```python
from build123d import *

# Parameters (mm, degrees)
F1_DEPTH = 20
F3_DEPTH = 0.2
F5_DEPTH = 20.001


with BuildPart() as f1:
    # F0 (on Top) → F1 (new body)
    with BuildSketch(Plane.XY):
        with BuildLine():
            Line((8, 10), (-8, 10))
            ThreePointArc((-8, 10), (-9.414214, 9.414214), (-10, 8))
            Line((-10, 8), (-10, -8))
            ThreePointArc((-10, -8), (-9.414214, -9.414214), (-8, -10))
            Line((-8, -10), (8, -10))
            ThreePointArc((8, -10), (9.414214, -9.414214), (10, -8))
            Line((10, -8), (10, 8))
            ThreePointArc((10, 8), (9.414214, 9.414214), (8, 10))
        make_face()
    extrude(amount=F1_DEPTH)

    # F2 (on face) → F3 (join)
    with BuildSketch(Plane(origin=(0, 0, 0), x_dir=(1, 0, 0), z_dir=(0, 0, -1))):
        with BuildLine():
            Line((15, 20), (-15, 20))
            ThreePointArc((-15, 20), (-18.535534, 18.535534), (-20, 15))
            Line((-20, 15), (-20, -15))
            ThreePointArc((-20, -15), (-18.535534, -18.535534), (-15, -20))
            Line((-15, -20), (15, -20))
            ThreePointArc((15, -20), (18.535534, -18.535534), (20, -15))
            Line((20, -15), (20, 15))
            ThreePointArc((20, 15), (18.535534, 18.535534), (15, 20))
        make_face()
        with BuildLine():
            Line((8, -10), (-8, -10))
            ThreePointArc((-8, -10), (-9.414214, -9.414214), (-10, -8))
            Line((-10, -8), (-10, 8))
            ThreePointArc((-10, 8), (-9.414214, 9.414214), (-8, 10))
            Line((-8, 10), (8, 10))
            ThreePointArc((8, 10), (9.414214, 9.414214), (10, 8))
            Line((10, 8), (10, -8))
            ThreePointArc((10, -8), (9.414214, -9.414214), (8, -10))
        make_face(mode=Mode.SUBTRACT)
    extrude(amount=-F3_DEPTH)

    # F4 (on face) → F5 (cut, through all)
    with BuildSketch(Plane.XY.offset(20)):
        with BuildLine():
            ThreePointArc((-8, 9.2), (-8.848528, 8.848528), (-9.2, 8))
            Line((-9.2, 8), (-9.2, -8))
            ThreePointArc((-9.2, -8), (-8.848528, -8.848528), (-8, -9.2))
            Line((-8, -9.2), (8, -9.2))
            ThreePointArc((8, -9.2), (8.848528, -8.848528), (9.2, -8))
            Line((9.2, -8), (9.2, 8))
            ThreePointArc((9.2, 8), (8.848528, 8.848528), (8, 9.2))
            Line((8, 9.2), (-8, 9.2))
        make_face()
    extrude(amount=-F5_DEPTH, mode=Mode.SUBTRACT)


solid = f1.part
```
Design review of the part built by this model. Coordinates are the model's own, in mm. A direction names the side the tool comes from. Round coordinates to 2 decimals unless told otherwise and drop trailing zeros. Write each loop counter-clockwise with the first axis right and the second up, starting at its lowest first coordinate (ties: lowest second). Pieces come first, ordered by that corner, then holes.
Item 1: For faces 4 (the cylindrical face through (-8.839, 8.858, 10.14)), 5 (the flat face through (10, 0, 10)), 6 (the cylindrical face through (-9.43, -9.4, 9.96)), list the 3-axis set-ups (+Z, -Z, +X, -X, +Y, -Y) from which the entire face can be reached by the end or side of a thin tool; tool diameter is ignored.
Item 2: We need section C-C on z = 17.25. Write out the cut boundary in (x, y), and give its area (3 significant figures).
Item 3: The part is to be moulded in two halves that separate along Y. For faces 1 (the flat face through (9.2, 0, 10)), 2 (the cylindrical face through (-9.4, 9.43, 9.96)), 3 (the flat face through (-9, -9, 0)), say which applies: +Y half, -Y half, draft (parallel to the pull), parting line (faces both ways), or undercut.
Item 4: Clearance check with flat-ended pins moving along their axes: pin 1 Ø5 at (y, z) = (-2.5, 11.5) entering from +X; pin 2 Ø2 at (x, y) = (-9.5, 0) entering from -Z; pin 3 Ø6 at (y, z) = (13.5, 13) entering from +X; pin 4 Ø5 at (x, y) = (0.5, -16) entering from +Z. State where each tip first meets the part, or that it passes through.
Item 5: We need section A-A on x = -3.5. Write out the cut boundary in (y, z), and give its area (3 significant figures).
Item 6: We need section D-D on x = -12. Write out the cut boundary in (y, z).
Item 7: For probe 1 along Y at (x, z) = (-5.5, 8.5); probe 2 along Z at (x, y) = (-13, -10.5), list the stretches that pass through material, from the lowest coordinate up.
Returned:
1. face 4: +Z, -Z
1. face 5: +Z, +X, +Y, -Y
1. face 6: +Z, -X, -Y
2. outline: (-10, -8) arc R2 ccw to (-8, -10) - (8, -10) arc R2 ccw to (10, -8) - (10, 8) arc R2 ccw to (8, 10) - (-8, 10) arc R2 ccw to (-10, 8) - close; hole (-9.2, -8) arc R1.2 ccw to (-8, -9.2) - (8, -9.2) arc R1.2 ccw to (9.2, -8) - (9.2, 8) arc R1.2 ccw to (8, 9.2) - (-8, 9.2) arc R1.2 ccw to (-9.2, 8) - close
2. area: 59.2 mm2
3. face 1: undercut
3. face 2: +Y half
3. face 3: draft
4. pin 1: stops at x = 10
4. pin 2: stops at z = 0
4. pin 3: passes through
4. pin 4: stops at z = 0.2
5. outline: (-20, 0) - (-9.2, 0) - (-9.2, 20) - (-10, 20) - (-10, 0.2) - (-20, 0.2) - close; (9.2, 0) - (20, 0) - (20, 0.2) - (10, 0.2) - (10, 20) - (9.2, 20) - close
5. area: 36.0 mm2
6. outline: (-20, 0) - (20, 0) - (20, 0.2) - (-20, 0.2) - close
7. probe 1: y = -10 to -9.2, 9.2 to 10
7. probe 2: z = 0 to 0.2
